Autodesk Inventor part; units mm, degrees
ref_plane "C1_XY" through (0, 0, 0) normal (0, 0, 1) x (1, 0, 0)
ref_plane "C1_YZ" through (0, 0, 0) normal (1, 0, 0) x (0, 1, 0)
ref_plane "C1_ZX" through (0, 0, 0) normal (0, 1, 0) x (0, 0, 1)
sketch "Sketch_64" plane through (0, 0, 0) normal (0, 0, 1) x (1, 0, 0)
  line L0 (-10, -3) -> (-10, -9)
  arc A0 (-10, -9) -> (-9, -10) centre (-9, -9) ccw
  line L1 (-9, -10) -> (9, -10)
  arc A1 (9, -10) -> (10, -9) centre (9, -9) ccw
  line L2 (10, -9) -> (10, 9)
  arc A2 (10, 9) -> (9, 10) centre (9, 9) ccw
  line L3 (9, 10) -> (3, 10)
  line L4 (3, 10) -> (3, 8)
  line L5 (3, 8) -> (6, 8)
  line L6 (6, 8) -> (6, 7.0607)
  line L7 (6, 7.0607) -> (2.9393, 4)
  line L8 (2.9393, 4) -> (0.5196, 4)
  line L9 (0.5196, 4) -> (0, 3.7)
  line L10 (0, 3.7) -> (-0.5196, 4)
  line L11 (-0.5196, 4) -> (-2.9393, 4)
  line L12 (-2.9393, 4) -> (-6, 7.0607)
  line L13 (-6, 7.0607) -> (-6, 8)
  line L14 (-6, 8) -> (-3, 8)
  line L15 (-3, 8) -> (-3, 10)
  line L16 (-3, 10) -> (-9, 10)
  arc A3 (-9, 10) -> (-10, 9) centre (-9, 9) ccw
  line L17 (-10, 9) -> (-10, 3)
  line L18 (-10, 3) -> (-8, 3)
  line L19 (-8, 3) -> (-8, 6)
  line L20 (-8, 6) -> (-7.0607, 6)
  line L21 (-7.0607, 6) -> (-4, 2.9393)
  line L22 (-4, 2.9393) -> (-4, 0.5196)
  line L23 (-4, 0.5196) -> (-3.7, 0)
  line L24 (-3.7, 0) -> (-4, -0.5196)
  line L25 (-4, -0.5196) -> (-4, -2.9393)
  line L26 (-4, -2.9393) -> (-7.0607, -6)
  line L27 (-7.0607, -6) -> (-8, -6)
  line L28 (-8, -6) -> (-8, -3)
  line L29 (-8, -3) -> (-10, -3)
  line L30 (-6, -7.2678) -> (-6, -7.5)
  arc A4 (-6, -7.5) -> (-5.5, -8) centre (-5.5, -7.5) ccw
  line L31 (-5.5, -8) -> (7, -8)
  arc A5 (7, -8) -> (8, -7) centre (7, -7) ccw
  line L32 (8, -7) -> (8, 5.5)
  arc A6 (8, 5.5) -> (7.5, 6) centre (7.5, 5.5) ccw
  line L33 (7.5, 6) -> (7.2678, 6)
  arc A7 (7.2678, 6) -> (6.9142, 5.8536) centre (7.2678, 5.5) ccw
  line L34 (6.9142, 5.8536) -> (4.1464, 3.0858)
  arc A8 (4.1464, 3.0858) -> (4, 2.7322) centre (4.5, 2.7322) ccw
  line L35 (4, 2.7322) -> (4, -1)
  arc A9 (1, -4) -> (4, -1) centre (1, -1) ccw
  line L36 (1, -4) -> (-2.7322, -4)
  arc A10 (-2.7322, -4) -> (-3.0858, -4.1464) centre (-2.7322, -4.5) ccw
  line L37 (-3.0858, -4.1464) -> (-5.8536, -6.9142)
  arc A11 (-5.8536, -6.9142) -> (-6, -7.2678) centre (-5.5, -7.2678) ccw
extrude "Extrusion1" add sketch "Sketch_64" along normal mid plane 650
sketch "Sketch2" plane through (0, 0, 325) normal (0, 0, 1) x (-1, 0, 0)
  point P0 (0, 0)
hole "Hole1" at (0, 0, 325) direction (0, 0, -1) diameter 4.2 end through all both
ref_plane "C1_XY" through (0, 0, 0) normal (0, 0, 1) x (1, 0, 0)
ref_plane "C1_YZ" through (0, 0, 0) normal (1, 0, 0) x (0, 1, 0)
ref_plane "C1_ZX" through (0, 0, 0) normal (0, 1, 0) x (0, 0, 1)
thread "Thread1"
thread "Thread2"
properties part number "HFSTB5-2020-680" material "Aluminum 6061"
Geometry: final body of the model. Coordinates: model frame, mm. A direction names the side the tool comes from. Give positions to 0.01 mm unless a question says otherwise; leave off trailing zeros. Answer as CSV lines item,"result". Start each with the question number.
(1) Reachability of faces 1 (the face through (8, -1, -5)), 2 (the face through (10, 0, -5)) from +Z, -Z, +X, -X, +Y, -Y: full face, straight path, thin tool, end or side. Return the list, or none.
(2) Pin query (flat end, axial travel): P1, Ø1, axis at x = 1.5, z = 38.5, coming from the +Y side; P2, Ø2.5, axis at y = -1.5, z = 135, coming from the -X side; P3, Ø4, axis at x = 0, y = 0, coming from the +Z side. Return the tip coordinate at first contact, or that it passes through.
(3) Ray query, line 1 along Y through (x, z) = (0, -144.5); line 2 along X through (y, z) = (0, -40); line 3 along X through (y, z) = (-0.5, -169). Return the intervals inside material, ascending. Write a range as [from, to].
(4) Section query A-A (z = 60). Give the number of separate pieces and of enclosed holes in the cut face, and give its area (3 significant figures).
Worked answers:
1,face 1,"+Z, -Z"
1,face 2,"+Z, -Z, +X, +Y, -Y"
2,P1,"stops at y = 4"
2,P2,"stops at x = -4"
2,P3,"passes through"
3,line 1,"y = [-10, -8], [-4, -2.1], [2.1, 3.7]"
3,line 2,"x = [-3.7, -2.1], [2.1, 4], [8, 10]"
3,line 3,"x = [-3.99, -2.04], [2.04, 4], [8, 10]"
4,separate pieces,"1"
4,enclosed holes,"2"
4,area,"195 mm^2"
